```python
from build123d import *

# Parameters (mm, degrees)
SKETCH1_W           = 20
SKETCH1_H           = 6.2
BOSS_EXTRUDE1_DEPTH = 3
SNAP_START          = 0.3
SNAP_HOOK1_DEPTH    = 1.25
SNAP_START_2        = -2.157223338
SNAP_HOOK1_2_DEPTH  = 4.314446676
SNAP_START_3        = -2.366854455
SNAP_HOOK1_3_DEPTH  = 4.73370891
SNAP_START_4        = -2
SNAP_HOOK1_4_DEPTH  = 6
FILLET1_R           = 1
CUT_EXTRUDE1_REACH  = 14.594
SKETCH3_R           = 1.5
FILLET2_R           = 1


with BuildPart() as part:
    # Sketch1 → Boss-Extrude1 (new body)
    with BuildSketch(Plane.XY):
        Rectangle(SKETCH1_W, SKETCH1_H)
    extrude(amount=BOSS_EXTRUDE1_DEPTH)

    # Snap Hook1: read off the stored shape, not the designer's step
    # Snap Hook1 outline → Snap Hook1 (add)
    with BuildSketch(Plane(origin=(0, 0, 0), x_dir=(1, 0, 0), z_dir=(0, 1, 0)).offset(SNAP_START)):
        Polygon((2.366854455, -3), (-2.366854455, -3), (-2, -10), (2, -10), align=None)
    extrude(amount=SNAP_HOOK1_DEPTH)

    # Snap Hook1 2 outline → Snap Hook1 2 (add)
    with BuildSketch(Plane.YZ.offset(SNAP_START_2)):
        Polygon((0.3, 3), (0.3, 10), (-1.45, 3), align=None)
        Polygon((1.55, 10), (1.55, 7), (3.05, 7), (3.05, 8), align=None)
    extrude(amount=SNAP_HOOK1_2_DEPTH)

    # Snap Hook1 3 outline → Snap Hook1 3 (add)
    with BuildSketch(Plane.YZ.offset(SNAP_START_3)):
        Polygon((0.3, 3), (0.3, 10), (-1.45, 3), align=None)
    extrude(amount=SNAP_HOOK1_3_DEPTH)

    # Snap Hook1 4 outline → Snap Hook1 4 (cut)
    with BuildSketch(Plane(origin=(0, 0, 0), x_dir=(1, 0, 0), z_dir=(0, 1, 0)).offset(SNAP_START_4)):
        Polygon((-2.366854455, -3), (-2.366854455, -11), (-1.947592221, -11), (-2, -10), align=None)
        Polygon((2, -10), (1.947592221, -11), (2.366854455, -11), (2.366854455, -3), align=None)
    extrude(amount=SNAP_HOOK1_4_DEPTH, mode=Mode.SUBTRACT)

    # Fillet1
    # the kernel refuses this fillet: 1 mm, written as the material it adds along each edge
    with BuildSketch(Plane(origin=(4.866854455, 1.55, 3), x_dir=(0, 1, 0), z_dir=(-1, 0, 0))) as fillet1_piece_1_section:
        with BuildLine():
            CenterArc((FILLET1_R, -FILLET1_R), FILLET1_R, 90, 90)
            Line((0, -FILLET1_R), (0, 0))
            Line((0, 0), (FILLET1_R, 0))
        make_face()
    fillet1_piece_1 = extrude(amount=9.73370891, mode=Mode.PRIVATE)
    fillet1_piece_1 = split(fillet1_piece_1, bisect_by=Plane(origin=(-2.347040948, 1.55, 3.378064238), z_dir=(0.9986295347544344, 0, -0.05233595624560593)), keep=Keep.TOP, mode=Mode.PRIVATE)
    fillet1_piece_1 = split(fillet1_piece_1, bisect_by=Plane(origin=(2.373702086, 1.55, 2.869339421), z_dir=(-0.9986295347544344, 0, -0.05233595624560593)), keep=Keep.TOP, mode=Mode.PRIVATE)
    add(fillet1_piece_1)
    with BuildSketch(Plane(origin=(2.366854455, 1.55, 3), x_dir=(1, 0, 0), z_dir=(0, -1, 0))) as fillet1_piece_2_section:
        with BuildLine():
            CenterArc((FILLET1_R * 0.948964566712, FILLET1_R), FILLET1_R, 183, 87)
            Line((-FILLET1_R * 0.0496649680421, FILLET1_R * 0.947664043754), (0, 0))
            Line((0, 0), (FILLET1_R * 0.948964566712, 0))
        make_face()
    fillet1_piece_2 = extrude(amount=5.372411417, mode=Mode.PRIVATE)
    fillet1_piece_2 = split(fillet1_piece_2, bisect_by=Plane(origin=(2.366854455, -1.273529412, 3.705882353), z_dir=(0, 0.9701425001453319, -0.24253562503633297)), keep=Keep.TOP, mode=Mode.PRIVATE)
    add(fillet1_piece_2)
    with BuildSketch(Plane(origin=(4.318795471, -1.45, 3), x_dir=(0, -1, 0), z_dir=(-1, 0, 0))) as fillet1_piece_3_section:
        with BuildLine():
            CenterArc((FILLET1_R * 0.780776406404, FILLET1_R), FILLET1_R, 194.036243468, 75.963756532)
            Line((-FILLET1_R * 0.189366093741, FILLET1_R * 0.757464374964), (0, 0))
            Line((0, 0), (FILLET1_R * 0.780776406404, 0))
        make_face()
    fillet1_piece_3 = extrude(amount=8.637590942, mode=Mode.PRIVATE)
    fillet1_piece_3 = split(fillet1_piece_3, bisect_by=Plane(origin=(2.372200924, -1.45, 2.897983303), z_dir=(-0.9986295347544344, 0, -0.05233595624560593)), keep=Keep.TOP, mode=Mode.PRIVATE)
    fillet1_piece_3 = split(fillet1_piece_3, bisect_by=Plane(origin=(-2.34854211, -1.45, 3.349420356), z_dir=(0.9986295347544344, 0, -0.05233595624560593)), keep=Keep.TOP, mode=Mode.PRIVATE)
    add(fillet1_piece_3)
    with BuildSketch(Plane(origin=(-2.366854455, -3.822411417, 3), x_dir=(-1, 0, 0), z_dir=(0, 1, 0))) as fillet1_piece_4_section:
        with BuildLine():
            CenterArc((FILLET1_R * 0.948964566712, FILLET1_R), FILLET1_R, 183, 87)
            Line((-FILLET1_R * 0.0496649680421, FILLET1_R * 0.947664043754), (0, 0))
            Line((0, 0), (FILLET1_R * 0.948964566712, 0))
        make_face()
    fillet1_piece_4 = extrude(amount=5.372411417, mode=Mode.PRIVATE)
    fillet1_piece_4 = split(fillet1_piece_4, bisect_by=Plane(origin=(-2.366854455, -1.589553613, 2.441785549), z_dir=(0, 0.9701425001453319, -0.24253562503633297)), keep=Keep.TOP, mode=Mode.PRIVATE)
    add(fillet1_piece_4)
    with BuildSketch(Plane(origin=(2.366854455, 3.922411417, 3), x_dir=(1, 0, 0), z_dir=(0, -1, 0))) as fillet1_piece_5a_section:
        with BuildLine():
            CenterArc((FILLET1_R * 0.948964566712, FILLET1_R), FILLET1_R, 183, 87)
            Line((-FILLET1_R * 0.0496649680421, FILLET1_R * 0.947664043754), (0, 0))
            Line((0, 0), (FILLET1_R * 0.948964566712, 0))
        make_face()
    fillet1_piece_5a = extrude(amount=7.744822834, mode=Mode.PRIVATE)
    fillet1_piece_5a = split(fillet1_piece_5a, bisect_by=Plane(origin=(2.366854455, 3.1, 3), z_dir=(0, -1, 0)), keep=Keep.TOP, mode=Mode.PRIVATE)
    fillet1_piece_5a = split(fillet1_piece_5a, bisect_by=Plane(origin=(2.366854455, 1.55, 3), z_dir=(0, 1, 0)), keep=Keep.TOP, mode=Mode.PRIVATE)
    with BuildSketch(Plane(origin=(4.866854455, 1.55, 3), x_dir=(0, 1, 0), z_dir=(-1, 0, 0))) as fillet1_piece_5b_section:
        with BuildLine():
            CenterArc((FILLET1_R, -FILLET1_R), FILLET1_R, 90, 90)
            Line((0, -FILLET1_R), (0, 0))
            Line((0, 0), (FILLET1_R, 0))
        make_face()
    fillet1_piece_5b = extrude(amount=9.73370891, mode=Mode.PRIVATE)
    fillet1_piece_5b = split(fillet1_piece_5b, bisect_by=Plane(origin=(2.373702086, 1.55, 2.869339421), z_dir=(0.9986295347544344, 0, 0.05233595624560593)), keep=Keep.TOP, mode=Mode.PRIVATE)
    fillet1_piece_5 = fillet1_piece_5a & fillet1_piece_5b
    add(fillet1_piece_5)
    with BuildSketch(Plane(origin=(4.866854455, 1.55, 3), x_dir=(0, 1, 0), z_dir=(-1, 0, 0))) as fillet1_piece_6a_section:
        with BuildLine():
            CenterArc((FILLET1_R, -FILLET1_R), FILLET1_R, 90, 90)
            Line((0, -FILLET1_R), (0, 0))
            Line((0, 0), (FILLET1_R, 0))
        make_face()
    fillet1_piece_6a = extrude(amount=9.73370891, mode=Mode.PRIVATE)
    fillet1_piece_6a = split(fillet1_piece_6a, bisect_by=Plane(origin=(-2.347040948, 1.55, 3.378064238), z_dir=(-0.9986295347544344, 0, 0.05233595624560593)), keep=Keep.TOP, mode=Mode.PRIVATE)
    with BuildSketch(Plane(origin=(-2.366854455, -3.822411417, 3), x_dir=(-1, 0, 0), z_dir=(0, 1, 0))) as fillet1_piece_6b_section:
        with BuildLine():
            CenterArc((FILLET1_R * 0.948964566712, FILLET1_R), FILLET1_R, 183, 87)
            Line((-FILLET1_R * 0.0496649680421, FILLET1_R * 0.947664043754), (0, 0))
            Line((0, 0), (FILLET1_R * 0.948964566712, 0))
        make_face()
    fillet1_piece_6b = extrude(amount=7.744822834, mode=Mode.PRIVATE)
    fillet1_piece_6b = split(fillet1_piece_6b, bisect_by=Plane(origin=(-2.366854455, 3.1, 3), z_dir=(0, -1, 0)), keep=Keep.TOP, mode=Mode.PRIVATE)
    fillet1_piece_6b = split(fillet1_piece_6b, bisect_by=Plane(origin=(-2.366854455, 1.55, 3), z_dir=(0, 1, 0)), keep=Keep.TOP, mode=Mode.PRIVATE)
    fillet1_piece_6 = fillet1_piece_6a & fillet1_piece_6b
    add(fillet1_piece_6)
    with BuildSketch(Plane(origin=(2.366854455, 1.55, 3), x_dir=(1, 0, 0), z_dir=(0, -1, 0))) as fillet1_piece_7a_section:
        with BuildLine():
            CenterArc((FILLET1_R * 0.948964566712, FILLET1_R), FILLET1_R, 183, 87)
            Line((-FILLET1_R * 0.0496649680421, FILLET1_R * 0.947664043754), (0, 0))
            Line((0, 0), (FILLET1_R * 0.948964566712, 0))
        make_face()
    fillet1_piece_7a = extrude(amount=5.372411417, mode=Mode.PRIVATE)
    fillet1_piece_7a = split(fillet1_piece_7a, bisect_by=Plane(origin=(2.366854455, -3.1, 3), z_dir=(0, 1, 0)), keep=Keep.TOP, mode=Mode.PRIVATE)
    fillet1_piece_7a = split(fillet1_piece_7a, bisect_by=Plane(origin=(2.366854455, -1.273529412, 3.705882353), z_dir=(0, -0.9701425001453319, 0.24253562503633297)), keep=Keep.TOP, mode=Mode.PRIVATE)
    with BuildSketch(Plane(origin=(4.318795471, -1.45, 3), x_dir=(0, -1, 0), z_dir=(-1, 0, 0))) as fillet1_piece_7b_section:
        with BuildLine():
            CenterArc((FILLET1_R * 0.780776406404, FILLET1_R), FILLET1_R, 194.036243468, 75.963756532)
            Line((-FILLET1_R * 0.189366093741, FILLET1_R * 0.757464374964), (0, 0))
            Line((0, 0), (FILLET1_R * 0.780776406404, 0))
        make_face()
    fillet1_piece_7b = extrude(amount=8.637590942, mode=Mode.PRIVATE)
    fillet1_piece_7b = split(fillet1_piece_7b, bisect_by=Plane(origin=(2.372200924, -1.45, 2.897983303), z_dir=(0.9986295347544344, 0, 0.05233595624560593)), keep=Keep.TOP, mode=Mode.PRIVATE)
    fillet1_piece_7 = fillet1_piece_7a & fillet1_piece_7b
    add(fillet1_piece_7)
    with BuildSketch(Plane(origin=(-2.366854455, -3.822411417, 3), x_dir=(-1, 0, 0), z_dir=(0, 1, 0))) as fillet1_piece_8a_section:
        with BuildLine():
            CenterArc((FILLET1_R * 0.948964566712, FILLET1_R), FILLET1_R, 183, 87)
            Line((-FILLET1_R * 0.0496649680421, FILLET1_R * 0.947664043754), (0, 0))
            Line((0, 0), (FILLET1_R * 0.948964566712, 0))
        make_face()
    fillet1_piece_8a = extrude(amount=5.372411417, mode=Mode.PRIVATE)
    fillet1_piece_8a = split(fillet1_piece_8a, bisect_by=Plane(origin=(-2.366854455, -3.1, 3), z_dir=(0, 1, 0)), keep=Keep.TOP, mode=Mode.PRIVATE)
    fillet1_piece_8a = split(fillet1_piece_8a, bisect_by=Plane(origin=(-2.366854455, -1.589553613, 2.441785549), z_dir=(0, -0.9701425001453319, 0.24253562503633297)), keep=Keep.TOP, mode=Mode.PRIVATE)
    with BuildSketch(Plane(origin=(4.318795471, -1.45, 3), x_dir=(0, -1, 0), z_dir=(-1, 0, 0))) as fillet1_piece_8b_section:
        with BuildLine():
            CenterArc((FILLET1_R * 0.780776406404, FILLET1_R), FILLET1_R, 194.036243468, 75.963756532)
            Line((-FILLET1_R * 0.189366093741, FILLET1_R * 0.757464374964), (0, 0))
            Line((0, 0), (FILLET1_R * 0.780776406404, 0))
        make_face()
    fillet1_piece_8b = extrude(amount=8.637590942, mode=Mode.PRIVATE)
    fillet1_piece_8b = split(fillet1_piece_8b, bisect_by=Plane(origin=(-2.34854211, -1.45, 3.349420356), z_dir=(-0.9986295347544344, 0, 0.05233595624560593)), keep=Keep.TOP, mode=Mode.PRIVATE)
    fillet1_piece_8 = fillet1_piece_8a & fillet1_piece_8b
    add(fillet1_piece_8)

    # Sketch3 → Cut-Extrude1 (cut, up to next)
    with BuildSketch(Plane.XY.offset(3), mode=Mode.PRIVATE) as cut_extrude1_sk1:
        with Locations((-6.657909511, 0)):
            Circle(SKETCH3_R)
    cut_extrude1_tool1 = extrude(cut_extrude1_sk1.sketch, amount=-CUT_EXTRUDE1_REACH, mode=Mode.PRIVATE) & part.part
    cut_extrude1 = cut_extrude1_tool1.solids().sort_by_distance((-6.65791, 0, 3))[0]
    add(cut_extrude1, mode=Mode.SUBTRACT)

    # Mirror1: Cut-Extrude1 across plane
    add(cut_extrude1.mirror(Plane(origin=(0, 0, 0), x_dir=(0, 0, 1), z_dir=(1, 0, 0))), mode=Mode.SUBTRACT)

    # Fillet2
    fillet2_edges = [part.edges().sort_by_distance(p)[0] for p in [
        (10, -3.1, 1.5),
        (-10, -3.1, 1.5),
        (-10, 3.1, 1.5),
        (10, 3.1, 1.5),
    ]]
    fillet(fillet2_edges, radius=FILLET2_R)


solid = part.part
```
Verification items for the finished model (mm, model axes). A direction names the side the tool comes from. Coordinates: 2 decimals unless noted, no trailing zeros. Loops run counter-clockwise (first coordinate to the right, second up) from the corner with the lowest first, then second, coordinate; pieces in that order, holes last. Notation, with made-up numbers: (-22.75, 88.5) - (1.25, 88.5) arc R34 cw to (1.25, 120.5) - close; hole circle Ø1 at (13, 28.5). An arc over 180 degrees is marked (long way). Answer as a JSON object with one key per item and string values.
(1) Cross-section at A-A, the plane z = 2.75. Record the boundary of the cut face in (x, y), then the cut area to 3 significant figures.
Response:
{"outline": "(-10, -2.1) arc R1 ccw to (-9, -3.1) - (9, -3.1) arc R1 ccw to (10, -2.1) - (10, 2.1) arc R1 ccw to (9, 3.1) - (-9, 3.1) arc R1 ccw to (-10, 2.1) - close; hole circle Ø3 at (-6.66, 0); hole circle Ø3 at (6.66, 0)", "area": "109 mm²"}
(2) Scan lines: line 1 along X through (y, z) = (0, 8); line 2 along Z through (x, y) = (9, -1.25); line 3 along X through (y, z) = (0.75, 7). Record each from-to range of solid material in increasing order.
Response:
{"line 1": "x = -2.1 to 2.1", "line 2": "z = 0 to 3", "line 3": "x = -2.16 to 2.16"}
(3) Cross-section at D-D, the plane y = -2.5. Record the boundary of the cut face in (x, z).
Response:
{"outline": "(-9.92, 0) - (9.92, 0) - (9.92, 3) - (-9.92, 3) - close"}
(4) Cross-section at B-B, the plane y = -1. Record the boundary of the cut face in (x, z), then the cut area to 3 significant figures.
Response:
{"outline": "(-10, 0) - (-7.78, 0) - (-7.78, 3) - (-10, 3) - close; (-5.54, 0) - (5.54, 0) - (5.54, 3) - (3.32, 3) arc R1 cw to (2.32, 3.95) - (2.27, 4.8) - (-2.27, 4.8) - (-2.32, 3.95) arc R1 cw to (-3.32, 3) - (-5.54, 3) - close; (7.78, 0) - (10, 0) - (10, 3) - (7.78, 3) - close", "area": "55.3 mm²"}
(5) Go/stop test with flat-tipped pins: pin 1 Ø2.5 at (x, y) = (-6.66, 0) entering from +Z; pin 2 Ø2 at (y, z) = (1.5, 4.5) entering from +X; pin 3 Ø1 at (x, z) = (-2, 5.5) entering from +Y; pin 4 Ø0.8 at (x, z) = (0, 7.5) entering from +Y. Record where each tip stops, or that it passes through.
Response:
{"pin 1": "passes through", "pin 2": "stops at x = 2.45", "pin 3": "stops at y = 1.55", "pin 4": "stops at y = 3.05"}
(6) Mould release check, pull along Y, two halves, no side actions. Record for faces 1 (the flat face through (0, -3.1, 1)), 2 (the cylindrical face through (-5.27, -0.57, 1.52)), 3 (the flat face through (-10, 0, 1)), 4 (the cylindrical face through (9.699, 2.815, 1.521)): pulls with the +Y half, pulls with the -Y half, needs draft (parallel to the pull), parting line crosses it, or undercut.
Response:
{"face 1": "pulls with the -Y half", "face 2": "undercut", "face 3": "needs draft", "face 4": "pulls with the +Y half"}
(7) Access from +Z, -Z, +X, -X, +Y, -Y to the whole of each face (thin tool, end or side, straight path). Record for faces 5 (the flat face through (0, 3.05, 7.5)), 6 (the cylindrical face through (-2.75, 0.126, 3.175)).
Response:
{"face 5": "+Z, +X, -X, +Y", "face 6": "+Z, -X, +Y, -Y"}
(8) Cross-section at C-C, the plane x = -3. Record the boundary of the cut face in (y, z), then the cut area to 3 significant figures.
Response:
{"outline": "(-3.1, 0) - (3.1, 0) - (3.1, 3) - (2.55, 3) arc R1 cw to (2.23, 3.05) - (-1.91, 3.05) arc R1 cw to (-2.23, 3) - (-3.1, 3) - close", "area": "18.8 mm²"}
